from build123d import *

# Parameters (mm, degrees)
SKETCH1_W           = 200
SKETCH1_H           = 100
BOSS_EXTRUDE1_DEPTH = 5
SKETCH2_W           = 200
SKETCH2_H           = 5
BOSS_EXTRUDE2_DEPTH = 50
SKETCH3_R           = 1.75
CUT_EXTRUDE1_DEPTH  = 50
SKETCH4_R           = 2.5
CUT_EXTRUDE2_DEPTH  = 123.474487139
SKETCH7_R           = 2
CUT_EXTRUDE3_DEPTH  = 123.474487139
SKETCH8_R           = 1.75
CUT_EXTRUDE4_DEPTH  = 123.474487139
SKETCH11_R          = 5
CUT_EXTRUDE6_DEPTH  = 149.492424049
SKETCH12_R          = 1.75
CUT_EXTRUDE7_DEPTH  = 123.474487139


with BuildPart() as part:
    # Sketch1 → Boss-Extrude1 (new body)
    with BuildSketch(Plane(origin=(0, 0, 0), x_dir=(1, 0, 0), z_dir=(0, 1, 0))):
        Rectangle(SKETCH1_W, SKETCH1_H)
    extrude(amount=BOSS_EXTRUDE1_DEPTH)

    # Sketch2 → Boss-Extrude2 (add)
    with BuildSketch(Plane(origin=(0, 5, 0), x_dir=(1, 0, 0), z_dir=(0, 1, 0))):
        with Locations((0, 47.5)):
            Rectangle(SKETCH2_W, SKETCH2_H)
    extrude(amount=BOSS_EXTRUDE2_DEPTH)

    # Sketch3 → Cut-Extrude1 (cut)
    with BuildSketch(Plane(origin=(0, 0, -50), x_dir=(-1, 0, 0), z_dir=(0, 0, -1))):
        with Locations((-93, 39)):
            Circle(SKETCH3_R)
        with Locations((-56, 12)):
            Circle(SKETCH3_R)
    extrude(amount=-CUT_EXTRUDE1_DEPTH, mode=Mode.SUBTRACT)

    # Sketch4 → Cut-Extrude2 (cut, through all)
    with BuildSketch(Plane(origin=(0, 5, 0), x_dir=(1, 0, 0), z_dir=(0, 1, 0))):
        with Locations(Location((28.85, 5, 0), (0, 0, 270))):
            Circle(SKETCH4_R)
        with Locations(Location((89, 5, 0), (0, 0, 270))):
            Circle(SKETCH4_R)
    extrude(amount=-CUT_EXTRUDE2_DEPTH, mode=Mode.SUBTRACT)

    # Sketch7 → Cut-Extrude3 (cut, through all)
    with BuildSketch(Plane(origin=(0, 5, 0), x_dir=(1, 0, 0), z_dir=(0, 1, 0))):
        with Locations(Location((-93, 17, 0), (0, 0, 270))):
            Circle(SKETCH7_R)
        with Locations(Location((-33, 17, 0), (0, 0, 270))):
            Circle(SKETCH7_R)
        with Locations(Location((-33, -43, 0), (0, 0, 270))):
            Circle(SKETCH7_R)
        with Locations(Location((-93, -43, 0), (0, 0, 270))):
            Circle(SKETCH7_R)
    extrude(amount=-CUT_EXTRUDE3_DEPTH, mode=Mode.SUBTRACT)

    # Sketch8 → Cut-Extrude4 (cut, through all)
    with BuildSketch(Plane(origin=(0, 5, 0), x_dir=(1, 0, 0), z_dir=(0, 1, 0))):
        with Locations(Location((65.125, -38.08, 0), (0, 0, 270))):
            Circle(SKETCH8_R)
        with Locations(Location((34.875, -21.92, 0), (0, 0, 270))):
            Circle(SKETCH8_R)
    extrude(amount=-CUT_EXTRUDE4_DEPTH, mode=Mode.SUBTRACT)

    # Sketch11 → Cut-Extrude6 (cut, through all)
    with BuildSketch(Plane.XY.offset(-45)):
        with Locations((-75.980762114, 20)):
            Circle(SKETCH11_R)
        with Locations((-50, 35)):
            Circle(SKETCH11_R)
        with Locations((-24.019237886, 20)):
            Circle(SKETCH11_R)
        with BuildLine():
            Line((-87.717456708, 22.5), (-85.717456708, 22.073985677))
            ThreePointArc((-85.717456708, 22.073985677), (-85.935893364, 20), (-85.717456708, 17.926014323))
            Line((-85.717456708, 17.926014323), (-87.717456708, 17.5))
            ThreePointArc((-87.717456708, 17.5), (-87.980762114, 20), (-87.717456708, 22.5))
        make_face()
        with BuildLine():
            Line((-40.263305406, 37.073985677), (-38.263305406, 37.5))
            ThreePointArc((-38.263305406, 37.5), (-38, 35), (-38.263305406, 32.5))
            Line((-38.263305406, 32.5), (-40.263305406, 32.926014323))
            ThreePointArc((-40.263305406, 32.926014323), (-40.04486875, 35), (-40.263305406, 37.073985677))
        make_face()
        with BuildLine():
            Line((-35.755932481, 22.5), (-33.755932481, 22.073985677))
            ThreePointArc((-33.755932481, 22.073985677), (-33.974369137, 20), (-33.755932481, 17.926014323))
            Line((-33.755932481, 17.926014323), (-35.755932481, 17.5))
            ThreePointArc((-35.755932481, 17.5), (-36.019237886, 20), (-35.755932481, 22.5))
        make_face()
    extrude(amount=-CUT_EXTRUDE6_DEPTH, mode=Mode.SUBTRACT)

    # Sketch12 → Cut-Extrude7 (cut, through all)
    with BuildSketch(Plane(origin=(0, 5, 0), x_dir=(1, 0, 0), z_dir=(0, 1, 0))):
        with Locations(Location((-9, 41, 0), (0, 0, 270))):
            Circle(SKETCH12_R)
        with Locations(Location((45, 41, 0), (0, 0, 270))):
            Circle(SKETCH12_R)
        with Locations(Location((-9, 17, 0), (0, 0, 270))):
            Circle(SKETCH12_R)
        with Locations(Location((45, 17, 0), (0, 0, 270))):
            Circle(SKETCH12_R)
    extrude(amount=-CUT_EXTRUDE7_DEPTH, mode=Mode.SUBTRACT)


solid = part.part
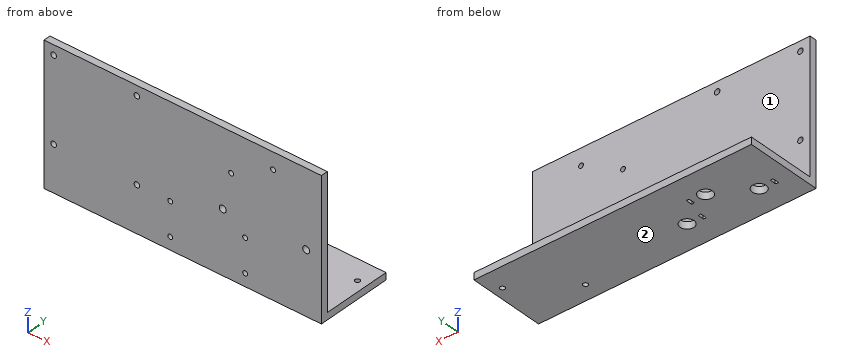
Model file for the job. Use its own axes, mm. Face numbers are marked on the shaded views. A direction names the side the tool comes from. Give positions to 0.01 mm unless a question says otherwise; leave off trailing zeros. Loops run counter-clockwise (first coordinate to the right, second up) from the corner with the lowest first, then second, coordinate; pieces in that order, holes last.
1) Wall check: line 1 (X direction, y = 1.6, z = -17); line 2 (X direction, y = 2, z = -41); line 3 (Y direction, x = 56, z = -47). Give the ranges that are in metal, low to high.
2) Flat gauge pins, fed straight in: pin 1 Ø4.5 at (x, z) = (34.875, 21.92) entering from +Y; pin 2 Ø15 at (x, y) = (-9.5, 39.5) entering from +Z. Where does each tip first touch, or does it go through?
3) Saw through at A-A (z = 43). Write the cut outline in (x, y), plus the area to 3 significant figures.
4) Saw through at C-C (x = -93). Write the cut outline in (y, z).
5) Saw through at B-B (y = 20). Write the cut outline in (x, z).
6) Saw through at D-D (y = 35). Write the cut outline in (x, z), plus the area to 3 significant figures.
7) Tool access for the marked faces 1 and 2: list every direction of +Z, -Z, +X, -X, +Y, -Y with a clear straight run to the whole face (end or side of a thin tool).
Answer block:
1. line 1: x = -100 to -95, -91 to -35, -31 to -10.75, -7.25 to 43.25, 46.75 to 100
1. line 2: x = -100 to -10.75, -7.25 to 43.25, 46.75 to 100
1. line 3: y = 0 to 10.25, 13.75 to 55
2. pin 1: stops at y = 5
2. pin 2: stops at z = -45
3. outline: (-100, 0) - (-95, 0) - (-95, 5) - (-100, 5) - close; (-91, 0) - (-35, 0) - (-35, 5) - (-91, 5) - close; (-31, 0) - (100, 0) - (100, 5) - (-31, 5) - close
3. area: 960 mm2
4. outline: (0, -50) - (55, -50) - (55, -45) - (5, -45) - (5, -19) - (0, -19) - close; (0, -15) - (5, -15) - (5, 41) - (0, 41) - close; (0, 45) - (5, 45) - (5, 50) - (0, 50) - close
5. outline: (-100, -50) - (-87.98, -50) - (-87.98, -45) - (-100, -45) - close; (-85.94, -50) - (-80.98, -50) - (-80.98, -45) - (-85.94, -45) - close; (-70.98, -50) - (-36.02, -50) - (-36.02, -45) - (-70.98, -45) - close; (-33.97, -50) - (-29.02, -50) - (-29.02, -45) - (-33.97, -45) - close; (-19.02, -50) - (100, -50) - (100, -45) - (-19.02, -45) - close
6. outline: (-100, -50) - (-55, -50) - (-55, -45) - (-100, -45) - close; (-45, -50) - (-40.04, -50) - (-40.04, -45) - (-45, -45) - close; (-38, -50) - (100, -50) - (100, -45) - (-38, -45) - close
6. area: 940 mm2
7. face 1: +Z, +X, -X, +Y
7. face 2: -Z, +X, -X, +Y, -Y
